Input: part model. Units: mm. Frame: model coordinates. A direction names the side the tool comes from. Coordinates: 2 decimals unless noted, no trailing zeros. Write each loop counter-clockwise with the first axis right and the second up, starting at its lowest first coordinate (ties: lowest second). Pieces come first, ordered by that corner, then holes. Notation, with made-up numbers: M 39.5,86 L 63.5,86 A17 cw 63.5,94 Z; hole C 6.5,81.5 d6. An arc over 180 degrees is marked long. Use CSV: the item, a comma, the result in double quotes.
```python
from build123d import *

# Parameters (mm, degrees)
SKETCH1_W                = 50
SKETCH1_H                = 50
BOSS_EXTRUDE1_DEPTH      = 50
CUT_EXTRUDE3_DEPTH       = 87.602540378
CUT_EXTRUDE4_DEPTH       = 87.602540378
CHAMFER1_SIZE            = 1.5
BOSS_EXTRUDE2_DEPTH      = 7
BOSS_EXTRUDE2_DEPTH_BACK = 10
SKETCH10_W               = 1
SKETCH10_H               = 7
SKETCH11_W               = 1.8
SKETCH11_H               = 1.8
CUT_EXTRUDE5_DEPTH       = 7


with BuildPart() as part:
    # Sketch1 → Boss-Extrude1 (new body)
    with BuildSketch(Plane.XY):
        with Locations((25, 25)):
            Rectangle(SKETCH1_W, SKETCH1_H)
    extrude(amount=BOSS_EXTRUDE1_DEPTH)

    # Sketch2 → Cut-Extrude3 (cut, through all)
    with BuildSketch(Plane.ZX):
        Polygon((61, 29.556349186), (54.556349186, 36), (45.443650814, 36), (39, 29.556349186), (39, 20.443650814), (45.443650814, 14), (54.556349186, 14), (61, 20.443650814), align=None)
    extrude(amount=CUT_EXTRUDE3_DEPTH, mode=Mode.SUBTRACT)

    # Sketch6 → Cut-Extrude4 (cut, through all)
    with BuildSketch(Plane(origin=(0, 0, 0), x_dir=(0, 0, -1), z_dir=(1, 0, 0))):
        Polygon((-61, 29.556349186), (-61, 20.443650814), (-54.556349186, 14), (-45.443650814, 14), (-39, 20.443650814), (-39, 29.556349186), (-45.443650814, 36), (-54.556349186, 36), align=None)
    extrude(amount=CUT_EXTRUDE4_DEPTH, mode=Mode.SUBTRACT)

    # Cut-Sweep5: sweep along a path in Sketch9
    with BuildLine(Plane(origin=(0, 25, 0), x_dir=(-1, 0, 0), z_dir=(0, -1, 0))) as cut_sweep5_path:
        Line((-50, -13.5), (-47, -13.5))
        ThreePointArc((-47, -13.5), (-31.443650814, -19.943650814), (-25, -35.5))
        Line((-25, -35.5), (-25, -50))
    # Sketch8 → Cut-Sweep5 (sweep, cut)
    with BuildSketch(Plane(origin=(50, 0, 0), x_dir=(0, 0, -1), z_dir=(1, 0, 0))):
        Polygon((-2.5, 29.556349186), (-8.943650814, 36), (-18.056349186, 36), (-24.5, 29.556349186), (-24.5, 20.443650814), (-18.056349186, 14), (-8.943650814, 14), (-2.5, 20.443650814), align=None)
    sweep(path=cut_sweep5_path.line, mode=Mode.SUBTRACT)

    # Chamfer1
    chamfer1_edges = [part.edges().sort_by_distance(p)[0] for p in [
        (50, 7, 50),
        (43, 50, 50),
        (43, 0, 50),
        (7, 50, 50),
        (14, 43, 50),
        (36, 7, 50),
        (36, 0, 47.721825407),
        (14, 0, 47.721825407),
        (14, 50, 47.721825407),
        (36, 50, 47.721825407),
        (32.778174593, 50, 42.221825407),
        (17.221825407, 50, 42.221825407),
        (32.778174593, 0, 42.221825407),
        (17.221825407, 0, 42.221825407),
        (0, 43, 50),
        (25, 50, 0),
        (50, 25, 0),
        (14, 7, 50),
        (36, 43, 50),
        (50, 43, 50),
        (25, 0, 0),
        (0, 7, 50),
        (0, 25, 0),
        (50, 36, 47.721825407),
        (50, 14, 47.721825407),
        (50, 17.221825407, 42.221825407),
        (50, 32.778174593, 42.221825407),
        (0, 14, 47.721825407),
        (0, 36, 47.721825407),
        (43, 14, 50),
        (7, 14, 50),
        (0, 17.221825407, 42.221825407),
        (0, 32.778174593, 42.221825407),
        (43, 36, 50),
        (7, 36, 50),
        (7, 0, 50),
        (0, 50, 25),
        (50, 50, 25),
        (50, 0, 25),
        (0, 0, 25),
    ]]
    chamfer(chamfer1_edges, length=CHAMFER1_SIZE)

    # Sketch10 → Boss-Extrude2 (add, two sides: drawn at the far end of the back side and taken through both)
    with BuildSketch(Plane.XY.offset(50).offset(-BOSS_EXTRUDE2_DEPTH_BACK)):
        with Locations((49.5, 7)):
            Rectangle(SKETCH10_W, SKETCH10_H)
    extrude(amount=BOSS_EXTRUDE2_DEPTH + BOSS_EXTRUDE2_DEPTH_BACK)

    # Sketch11 → Cut-Extrude5 (cut)
    with BuildSketch(Plane(origin=(50, 0, 0), x_dir=(0, 0, -1), z_dir=(1, 0, 0))):
        with Locations((-53.6, 7)):
            Rectangle(SKETCH11_W, SKETCH11_H)
    extrude(amount=-CUT_EXTRUDE5_DEPTH, mode=Mode.SUBTRACT)


solid = part.part
```
1. Section D-D (y = 5). Return loops of the section in (x, z).
Resolved:
outline,"M 0,1.5 L 1.5,0 L 48.5,0 L 50,1.5 L 50,57 L 49,57 L 49,49.5 L 48.5,50 L 37.5,50 L 36,48.5 L 36,45.44 L 29.56,39 L 20.44,39 L 14,45.44 L 14,48.5 L 12.5,50 L 1.5,50 L 0,48.5 Z"
2. Contact query for flat-ended pins moving along their axis: pin 1 Ø1 at (x, y) = (9, 44) entering from +Z; pin 2 Ø5.5 at (y, z) = (8, 51.5) entering from -X; pin 3 Ø14.5 at (x, y) = (22.5, 42) entering from +Z; pin 4 Ø2 at (x, z) = (12, 49) entering from -Y. Output: stop coordinate, or through.
Resolved:
pin 1,"stops at z = 50"
pin 2,"stops at x = 0.25"
pin 3,"stops at z = 44.19"
pin 4,"stops at y = 0"
3. Section B-B (y = 15.5). Return loops of the section in (x, z).
Resolved:
outline,"M 0,1.5 L 1.5,0 L 48.5,0 L 50,1.5 L 50,7.44 L 47,7.44 A28.06 cw 18.94,35.5 L 18.94,40.5 L 15.5,43.94 L 1.5,43.94 L 0,41.82 Z; M 31.06,35.5 A15.94 ccw 47,19.56 L 50,19.56 L 50,41.82 L 48.5,43.94 L 34.5,43.94 L 31.06,40.5 Z"
4. Section A-A (z = 47). Return loops of the section in (x, y), then the cut area to 4 significant figures.
Resolved:
outline,"M 0,1.5 L 1.5,0 L 12.5,0 L 14,1.5 L 14,14 L 1.5,14 L 0,12.5 Z; M 0,37.5 L 1.5,36 L 14,36 L 14,48.5 L 12.5,50 L 1.5,50 L 0,48.5 Z; M 36,1.5 L 37.5,0 L 48.5,0 L 50,1.5 L 50,12.5 L 48.5,14 L 36,14 Z; M 36,36 L 48.5,36 L 50,37.5 L 50,48.5 L 48.5,50 L 37.5,50 L 36,48.5 Z"
area,"770.5 mm^2"
5. Access query for faces 5 (the flat face through (17.177, 32.733, 38.161)), 6 (the flat face through (37, 49, 49)), 7 (the flat face through (49.2, 36.7, 46.6)), 8 (the flat face through (42.3, 13.3, 49.2)). Directions: +Z, -Z, +X, -X, +Y, -Y. A direction counts if a zero-diameter tool reaches every point of the face in a straight line with its end or side. Return the directions, or none.
Resolved:
face 5,"+Z"
face 6,"+Z, +Y"
face 7,"+Z, +X"
face 8,"+Z, +X, -X"
6. Material intervals for line 1 (Y direction, x = 38, z = 47); line 2 (Z direction, x = 11, y = 10.5); line 3 (X direction, y = 7.5, z = 44.5), sorted ascending. Write a range as [from, to].
Resolved:
line 1,"y = [0, 14], [36, 50]"
line 2,"z = [0, 50]"
line 3,"x = [0, 14.94], [35.06, 50]"
7. Section C-C (x = 8.5). Return loops of the section in (y, z), then the cut area to 3 significant figures.
Resolved:
outline,"M 0,1.5 L 1.5,0 L 48.5,0 L 50,1.5 L 50,48.5 L 48.5,50 L 37.5,50 L 36,48.5 L 36,45.44 L 29.56,39 L 20.44,39 L 14,45.44 L 14,48.5 L 12.5,50 L 1.5,50 L 0,48.5 Z"
area,"2,290 mm^2"
8. Mould query, pull axis Y, two halves, no side actions, for faces 1 (the flat face through (42, 14, 47)), 2 (the flat face through (36.7, 49.2, 46.6)), 3 (the flat face through (32.823, 17.267, 38.161)), 4 (the flat face through (43, 7, 50)). Classes: pulls with the +Y half, pulls with the -Y half, needs draft (parallel to the pull), parting line crosses it, or undercut.
Resolved:
face 1,"undercut"
face 2,"pulls with the +Y half"
face 3,"undercut"
face 4,"needs draft"
